from build123d import *

# Parameters (mm, degrees)
SZKIC1_R                    = 2
SZKIC1_R_2                  = 3
DODANIE_WYCI_GNI_CIE1_DEPTH = 2


with BuildPart() as part:
    # Szkic1 → Dodanie-wyciągnięcie1 (new body)
    with BuildSketch(Plane(origin=(0, 0, 0), x_dir=(1, 0, 0), z_dir=(0, 1, 0))):
        with BuildLine():
            Line((1700.559122815, -953.967589017), (1789.615327329, -887.395203569))
            ThreePointArc((1789.615327329, -887.395203569), (1792.419138662, -882.05438434), (1790.028740764, -876.516180127))
            Line((1790.028740764, -876.516180127), (1759.900801977, -850.204446919))
            ThreePointArc((1759.900801977, -850.204446919), (1754.293249598, -848.549066517), (1749.385441114, -851.726855661))
            Line((1749.385441114, -851.726855661), (1690.457175388, -944.610974317))
            ThreePointArc((1690.457175388, -944.610974317), (1691.611316681, -953.496529428), (1700.559122815, -953.967589017))
        make_face()
        with Locations((1755.296248665, -855.476836207)):
            Circle(SZKIC1_R, mode=Mode.SUBTRACT)
        with Locations((1785.424187453, -881.788569415)):
            Circle(SZKIC1_R, mode=Mode.SUBTRACT)
        with Locations((1696.367982939, -948.360954863)):
            Circle(SZKIC1_R_2, mode=Mode.SUBTRACT)
        with Locations((1709.760770604, -927.250927896)):
            Circle(SZKIC1_R_2, mode=Mode.SUBTRACT)
    extrude(amount=DODANIE_WYCI_GNI_CIE1_DEPTH)


solid = part.part
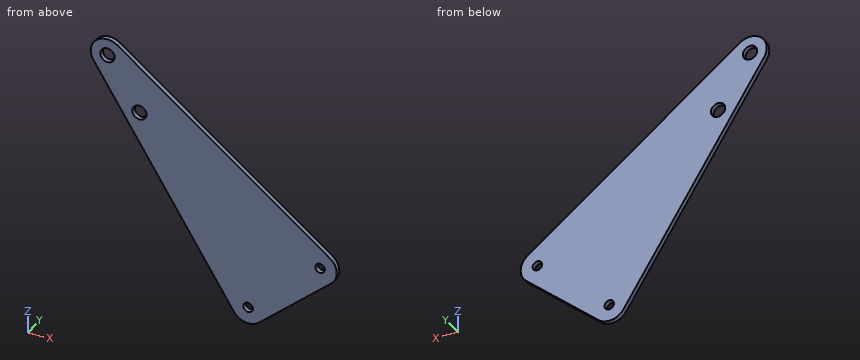
Here's how the part is built. I have some questions about the finished solid (model axes, mm). Coordinates: 2 decimals unless noted, no trailing zeros. Loops run counter-clockwise (first coordinate to the right, second up) from the corner with the lowest first, then second, coordinate; pieces in that order, holes last. Notation, with made-up numbers: (-10, 51.25) -> (4, 51.25) arc R17 cw to (4, 78.25) -> close; hole circle Ø4 at (-12, -12). An arc over 180 degrees is marked (long way). Use one line per item in the form item = value. Start each with the question number.
(1) If we section it at C-C (z = 860): Please give me the cut outline in (x, y).
(2) Please list where these lines run through material, in increasing order: line 1 along X through (y, z) = (1.05, 883.5); line 2 along Z through (x, y) = (1698, 0.8); line 3 along X through (y, z) = (0.35, 880.5).
(3) Will these pins go through, and if not, where does the flat tip stop? pin 1 (1 mm diameter, centred on x = 1708, z = 915.5, fed in from -Y); pin 2 (9.5 mm diameter, centred on x = 1696.37, z = 948.36, fed in from -Y).
(4) If we section it at A-A (y = 0.75): Please give me the cut outline in (x, z), then the cut area to 3 significant figures.
(5) If we section it at B-B (x = 1747): Please give me the cut outline in (y, z).
Verdict:
q1.outline = (1744.14, 0) -> (1771.12, 0) -> (1771.12, 2) -> (1744.14, 2) -> close
q2.line_1 = 1729.23 to 1784.39, 1786.46 to 1792.21
q2.line_2 = 932.72 to 945.84, 950.88 to 955.17
q2.line_3 = 1731.13 to 1783.89, 1786.95 to 1792.3
q3.pin_1 = through
q3.pin_2 = 0
q4.outline = (1690.46, 944.61) -> (1749.39, 851.73) arc R7 ccw to (1759.9, 850.2) -> (1790.03, 876.52) arc R7 ccw to (1789.62, 887.4) -> (1700.56, 953.97) arc R7 ccw to start; hole circle Ø6 at (1696.37, 948.36); hole circle Ø6 at (1709.76, 927.25); hole circle Ø4 at (1755.3, 855.48); hole circle Ø4 at (1785.42, 881.79)
q4.area = 4,080 mm²
q5.outline = (0, 855.49) -> (2, 855.49) -> (2, 919.25) -> (0, 919.25) -> close
